Part model, mm, in its own coordinate system. Face numbers are marked on the shaded views. A direction names the side the tool comes from. Round coordinates to 2 decimals unless told otherwise and drop trailing zeros. Write each loop counter-clockwise with the first axis right and the second up, starting at its lowest first coordinate (ties: lowest second). Pieces come first, ordered by that corner, then holes. Notation, with made-up numbers: M 77,30.25 L 125,30.25 A10 ccw 125,42.25 Z; hole C 73.5,27.5 d10. An arc over 180 degrees is marked long. One line per question, with ' | ' between items. Start each with the question number.
1) Drop flat-ended pins along their axis: pin 1 Ø5 at (y, z) = (4, -33.5) entering from +X; pin 2 Ø8 at (y, z) = (1, 32) entering from -X; pin 3 Ø9.5 at (x, z) = (38, -2) entering from +Y. Give the stop position or say it passes through.
2) Saw through at A-A (x = 0). List the corners of the cut face in (y, z), plus the area to 3 significant figures.
3) Saw through at B-B (z = 0). List the corners of the cut face in (x, y).
4) Tool access for the marked faces 1, 2, 3 and 4: list every direction of +Z, -Z, +X, -X, +Y, -Y with a clear straight run to the whole face (end or side of a thin tool).
5) Saw through at C-C (z = -19.5). List the corners of the cut face in (x, y), plus the area to 3 significant figures.
6) Mould opens along X. For the marked faces 5 and 6 say: pulls with the +X half, pulls with the -X half, needs draft (parallel to the pull), parting line crosses it, or undercut.
7) Wall check: probe 1 along X at (y, z) = (-1.5, -1); probe 2 along X at (y, z) = (7.5, 18); probe 3 along X at (y, z) = (10, 26). Give the ranges that are in metal, low to high. Write a range as [from, to].
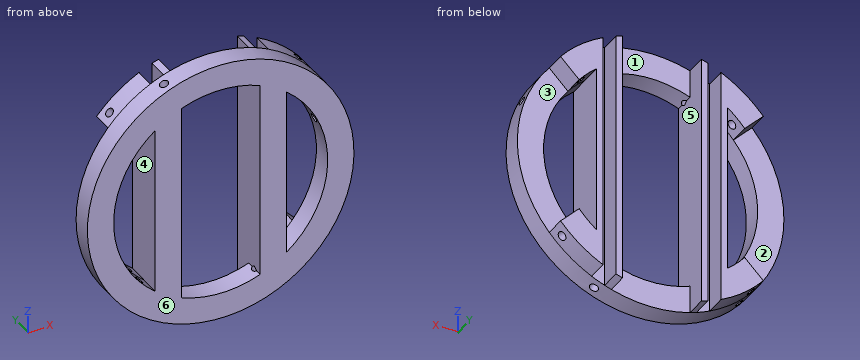
```python
from build123d import *
from build123d.topology import SkipClean

# Parameters (mm, degrees)
SKETCH1_R                       = 50.7746
BOSS_EXTRUDE1_DEPTH             = 4
BOSS_EXTRUDE2_START             = 8
BOSS_EXTRUDE2_DEPTH             = 8
M4_TAPPED_HOLE1_D               = 3.3
M4_TAPPED_HOLE1_DEPTH           = 10.1
M4_TAPPED_HOLE1_TIP             = 0.991420021
M4_TAPPED_HOLE1_ON_FACE_2_D     = 3.3
M4_TAPPED_HOLE1_ON_FACE_2_DEPTH = 10.1
M4_TAPPED_HOLE1_ON_FACE_2_TIP   = 0.991420021
M4_TAPPED_HOLE1_ON_FACE_3_D     = 3.3
M4_TAPPED_HOLE1_ON_FACE_3_DEPTH = 10.1
M4_TAPPED_HOLE1_ON_FACE_3_TIP   = 0.991420021
M4_TAPPED_HOLE1_ON_FACE_4_D     = 3.3
M4_TAPPED_HOLE1_ON_FACE_4_DEPTH = 10.1
M4_TAPPED_HOLE1_ON_FACE_4_TIP   = 0.991420021
M4_TAPPED_HOLE1_ON_FACE_5_D     = 3.3
M4_TAPPED_HOLE1_ON_FACE_5_DEPTH = 10.1
M4_TAPPED_HOLE1_ON_FACE_5_TIP   = 0.991420021
M4_TAPPED_HOLE1_ON_FACE_6_D     = 3.3
M4_TAPPED_HOLE1_ON_FACE_6_DEPTH = 10.1
M4_TAPPED_HOLE1_ON_FACE_6_TIP   = 0.991420021
M4_TAPPED_HOLE1_ON_FACE_7_D     = 3.3
M4_TAPPED_HOLE1_ON_FACE_7_DEPTH = 10.1
M4_TAPPED_HOLE1_ON_FACE_7_TIP   = 0.991420021
M4_TAPPED_HOLE1_ON_FACE_8_D     = 3.3
M4_TAPPED_HOLE1_ON_FACE_8_DEPTH = 10.1
M4_TAPPED_HOLE1_ON_FACE_8_TIP   = 0.991420021


with BuildPart() as part:
    # Sketch1 → Boss-Extrude1 (new, symmetric)
    with BuildSketch(Plane(origin=(0, 0, 0), x_dir=(1, 0, 0), z_dir=(0, 1, 0))):
        with Locations(Location((0, 0, 0), (0, 0, 270))):
            Circle(SKETCH1_R)
        with BuildLine():
            ThreePointArc((15, 37.915274035), (0, 40.7746), (-15, 37.915274035))
            Line((-15, 37.915274035), (-15, -37.915274035))
            ThreePointArc((-15, -37.915274035), (0, -40.7746), (15, -37.915274035))
            Line((15, -37.915274035), (15, 37.915274035))
        make_face(mode=Mode.SUBTRACT)
        with BuildLine():
            ThreePointArc((25, -32.211302444), (40.7746, 0), (25, 32.211302444))
            Line((25, 32.211302444), (25, -32.211302444))
        make_face(mode=Mode.SUBTRACT)
        with BuildLine():
            ThreePointArc((-25, 32.211302444), (-40.7746, 0), (-25, -32.211302444))
            Line((-25, -32.211302444), (-25, 32.211302444))
        make_face(mode=Mode.SUBTRACT)
    extrude(amount=BOSS_EXTRUDE1_DEPTH, both=True)

    # Sketch2 → Boss-Extrude2 (add)
    with SkipClean():  # the faces are left unmerged after this step: merging them gives an invalid solid
        with BuildSketch(Plane(origin=(0, 4, 0), x_dir=(1, 0, 0), z_dir=(0, 1, 0)).offset(BOSS_EXTRUDE2_START)):
            with BuildLine():
                Line((-22.5, -45.517139686), (-22.5, 45.517139686))
                ThreePointArc((-22.5, 45.517139686), (-31.197949015, 40.059305815), (-38.619906594, 32.963052344))
                Line((-38.619906594, 32.963052344), (-31.521353127, 25.864498878))
                ThreePointArc((-31.521353127, 25.864498878), (-28.438289659, 29.220398465), (-25, 32.211302444))
                Line((-25, 32.211302444), (-25, -32.211302444))
                ThreePointArc((-25, -32.211302444), (-28.438289659, -29.220398465), (-31.521353127, -25.864498878))
                Line((-31.521353127, -25.864498878), (-38.619906594, -32.963052344))
                ThreePointArc((-38.619906594, -32.963052344), (-31.197949015, -40.059305815), (-22.5, -45.517139686))
            make_face()
            with BuildLine():
                ThreePointArc((-15, 48.50834985), (-16.255489516, 48.102173192), (-17.5, 47.663508108))
                Line((-17.5, 47.663508108), (-17.5, -47.663508108))
                ThreePointArc((-17.5, -47.663508108), (-16.255489516, -48.102173192), (-15, -48.50834985))
                Line((-15, -48.50834985), (-15, 48.50834985))
            make_face()
            with BuildLine():
                ThreePointArc((17.5, 47.663508108), (16.255489516, 48.102173192), (15, 48.50834985))
                Line((15, 48.50834985), (15, -48.50834985))
                ThreePointArc((15, -48.50834985), (16.255489516, -48.102173192), (17.5, -47.663508108))
                Line((17.5, -47.663508108), (17.5, 47.663508108))
            make_face()
            with BuildLine():
                ThreePointArc((38.619906594, 32.963052344), (31.197949015, 40.059305815), (22.5, 45.517139686))
                Line((22.5, 45.517139686), (22.5, -45.517139686))
                ThreePointArc((22.5, -45.517139686), (31.197949015, -40.059305815), (38.619906594, -32.963052344))
                Line((38.619906594, -32.963052344), (31.521353127, -25.864498878))
                ThreePointArc((31.521353127, -25.864498878), (28.438289659, -29.220398465), (25, -32.211302444))
                Line((25, -32.211302444), (25, 32.211302444))
                ThreePointArc((25, 32.211302444), (28.438289659, 29.220398465), (31.521353127, 25.864498878))
                Line((31.521353127, 25.864498878), (38.619906594, 32.963052344))
            make_face()
        extrude(amount=-BOSS_EXTRUDE2_DEPTH)

    # M4 Tapped Hole1
    with Locations(Plane(origin=(-19.430598205, 0, 46.909613711), x_dir=(0.923879532511, 0, 0.382683432365), z_dir=(-0.382683432365, 0, 0.923879532511))):
        with Locations((0, 0)):
            Hole(M4_TAPPED_HOLE1_D / 2, depth=M4_TAPPED_HOLE1_DEPTH)
            with Locations((0, 0, -(M4_TAPPED_HOLE1_DEPTH + M4_TAPPED_HOLE1_TIP / 2))):  # 118° drill point
                Cone(0, M4_TAPPED_HOLE1_D / 2, M4_TAPPED_HOLE1_TIP, mode=Mode.SUBTRACT)

    # M4 Tapped Hole1 on face 2
    with Locations(Plane(origin=(46.909613711, 0, 19.430598205), x_dir=(-0.382682898036, 0, 0.923879753837), z_dir=(0.923879753837, 0, 0.382682898036))):
        with Locations((0, 0)):
            Hole(M4_TAPPED_HOLE1_ON_FACE_2_D / 2, depth=M4_TAPPED_HOLE1_ON_FACE_2_DEPTH)
            with Locations((0, 0, -(M4_TAPPED_HOLE1_ON_FACE_2_DEPTH + M4_TAPPED_HOLE1_ON_FACE_2_TIP / 2))):  # 118° drill point
                Cone(0, M4_TAPPED_HOLE1_ON_FACE_2_D / 2, M4_TAPPED_HOLE1_ON_FACE_2_TIP, mode=Mode.SUBTRACT)

    # M4 Tapped Hole1 on face 3
    with Locations(Plane(origin=(-35.903063972, 0, -35.903063972), x_dir=(-0.707106781187, 0, 0.707106781187), z_dir=(-0.707106781187, 0, -0.707106781187))):
        with Locations((0, 0), (0, 8)):
            Hole(M4_TAPPED_HOLE1_ON_FACE_3_D / 2, depth=M4_TAPPED_HOLE1_ON_FACE_3_DEPTH)
            with Locations((0, 0, -(M4_TAPPED_HOLE1_ON_FACE_3_DEPTH + M4_TAPPED_HOLE1_ON_FACE_3_TIP / 2))):  # 118° drill point
                Cone(0, M4_TAPPED_HOLE1_ON_FACE_3_D / 2, M4_TAPPED_HOLE1_ON_FACE_3_TIP, mode=Mode.SUBTRACT)

    # M4 Tapped Hole1 on face 4
    with Locations(Plane(origin=(19.430598205, 0, -46.909613711), x_dir=(-0.923879753837, 0, -0.382682898036), z_dir=(0.382682898036, 0, -0.923879753837))):
        with Locations((0, 0)):
            Hole(M4_TAPPED_HOLE1_ON_FACE_4_D / 2, depth=M4_TAPPED_HOLE1_ON_FACE_4_DEPTH)
            with Locations((0, 0, -(M4_TAPPED_HOLE1_ON_FACE_4_DEPTH + M4_TAPPED_HOLE1_ON_FACE_4_TIP / 2))):  # 118° drill point
                Cone(0, M4_TAPPED_HOLE1_ON_FACE_4_D / 2, M4_TAPPED_HOLE1_ON_FACE_4_TIP, mode=Mode.SUBTRACT)

    # M4 Tapped Hole1 on face 5
    with Locations(Plane(origin=(0, 8, 0), x_dir=(0.923879532511, 0, 0.382683432365), z_dir=(-0.382683432365, 0, 0.923879532511))):
        with Locations((0, 0)):
            Hole(M4_TAPPED_HOLE1_ON_FACE_5_D / 2, depth=M4_TAPPED_HOLE1_ON_FACE_5_DEPTH)
            with Locations((0, 0, -(M4_TAPPED_HOLE1_ON_FACE_5_DEPTH + M4_TAPPED_HOLE1_ON_FACE_5_TIP / 2))):  # 118° drill point
                Cone(0, M4_TAPPED_HOLE1_ON_FACE_5_D / 2, M4_TAPPED_HOLE1_ON_FACE_5_TIP, mode=Mode.SUBTRACT)

    # M4 Tapped Hole1 on face 6
    with Locations(Plane(origin=(35.903063972, 8, 35.903063972), x_dir=(0.707106781187, 0, -0.707106781187), z_dir=(0.707106781187, 0, 0.707106781187))):
        with Locations((0, 0)):
            Hole(M4_TAPPED_HOLE1_ON_FACE_6_D / 2, depth=M4_TAPPED_HOLE1_ON_FACE_6_DEPTH)
            with Locations((0, 0, -(M4_TAPPED_HOLE1_ON_FACE_6_DEPTH + M4_TAPPED_HOLE1_ON_FACE_6_TIP / 2))):  # 118° drill point
                Cone(0, M4_TAPPED_HOLE1_ON_FACE_6_D / 2, M4_TAPPED_HOLE1_ON_FACE_6_TIP, mode=Mode.SUBTRACT)

    # M4 Tapped Hole1 on face 7
    with Locations(Plane(origin=(35.903063972, 8, -35.903063972), x_dir=(-0.707106781187, 0, -0.707106781187), z_dir=(0.707106781187, 0, -0.707106781187))):
        with Locations((0, 0)):
            Hole(M4_TAPPED_HOLE1_ON_FACE_7_D / 2, depth=M4_TAPPED_HOLE1_ON_FACE_7_DEPTH)
            with Locations((0, 0, -(M4_TAPPED_HOLE1_ON_FACE_7_DEPTH + M4_TAPPED_HOLE1_ON_FACE_7_TIP / 2))):  # 118° drill point
                Cone(0, M4_TAPPED_HOLE1_ON_FACE_7_D / 2, M4_TAPPED_HOLE1_ON_FACE_7_TIP, mode=Mode.SUBTRACT)

    # M4 Tapped Hole1 on face 8
    with Locations(Plane(origin=(-35.903063972, 8, 35.903063972), x_dir=(0.707106781187, 0, 0.707106781187), z_dir=(-0.707106781187, 0, 0.707106781187))):
        with Locations((0, 0)):
            Hole(M4_TAPPED_HOLE1_ON_FACE_8_D / 2, depth=M4_TAPPED_HOLE1_ON_FACE_8_DEPTH)
            with Locations((0, 0, -(M4_TAPPED_HOLE1_ON_FACE_8_DEPTH + M4_TAPPED_HOLE1_ON_FACE_8_TIP / 2))):  # 118° drill point
                Cone(0, M4_TAPPED_HOLE1_ON_FACE_8_D / 2, M4_TAPPED_HOLE1_ON_FACE_8_TIP, mode=Mode.SUBTRACT)


solid = part.part
```
Answer key:
1) pin 1: stops at x = 40.21 | pin 2: stops at x = -42.36 | pin 3: stops at y = 4
2) outline: M -4,-50.77 L 4,-50.77 L 4,-40.77 L -4,-40.77 Z; M -4,40.77 L 4,40.77 L 4,50.77 L -4,50.77 Z | area: 160 mm2
3) outline: M -50.77,-4 L -40.77,-4 L -40.77,4 L -50.77,4 Z; M -25,-4 L -15,-4 L -15,12 L -17.5,12 L -17.5,4 L -22.5,4 L -22.5,12 L -25,12 Z; M 15,-4 L 25,-4 L 25,12 L 22.5,12 L 22.5,4 L 17.5,4 L 17.5,12 L 15,12 Z; M 40.77,-4 L 50.77,-4 L 50.77,4 L 40.77,4 Z
4) face 1: +Z, -Z, +Y | face 2: -X, +Y | face 3: +X, +Y | face 4: +Y, -Y
5) outline: M -46.88,-4 L -35.81,-4 L -35.81,4 L -46.88,4 Z; M -25,-4 L -15,-4 L -15,12 L -17.5,12 L -17.5,4 L -22.5,4 L -22.5,12 L -25,12 Z; M 15,-4 L 25,-4 L 25,12 L 22.5,12 L 22.5,4 L 17.5,4 L 17.5,12 L 15,12 Z; M 35.81,-4 L 46.88,-4 L 46.88,4 L 35.81,4 Z | area: 417 mm2
6) face 5: undercut | face 6: needs draft
7) probe 1: x = [-50.76, -40.76], [-25, -15], [15, 25], [40.76, 50.76] | probe 2: x = [-25, -22.5], [-17.5, -15], [15, 17.5], [22.5, 25] | probe 3: x = [-31.66, -31.41], [-25, -22.5], [-17.5, -15], [15, 17.5], [22.5, 25], [31.41, 31.66]
